```python
from build123d import *

# Parameters (mm, degrees)
SKETCH1_R           = 12.7
SKETCH1_R_2         = 2.4892
BOSS_EXTRUDE1_DEPTH = 0.79375


with BuildPart() as part:
    # Sketch1 → Boss-Extrude1 (new, symmetric)
    with BuildSketch(Plane(origin=(0, 0, 0), x_dir=(0, 0, -1), z_dir=(1, 0, 0))):
        with BuildLine():
            Line((-36.765056818, -4.392675398), (-7.053551136, -16.838589027))
            ThreePointArc((-7.053551136, -16.838589027), (0, -18.25625), (7.053551136, -16.838589027))
            Line((7.053551136, -16.838589027), (36.765056818, -4.392675398))
            ThreePointArc((36.765056818, -4.392675398), (39.6875, 0), (36.765056818, 4.392675398))
            Line((36.765056818, 4.392675398), (7.053551136, 16.838589027))
            ThreePointArc((7.053551136, 16.838589027), (0, 18.25625), (-7.053551136, 16.838589027))
            Line((-7.053551136, 16.838589027), (-36.765056818, 4.392675398))
            ThreePointArc((-36.765056818, 4.392675398), (-39.6875, 0), (-36.765056818, -4.392675398))
        make_face()
        Circle(SKETCH1_R, mode=Mode.SUBTRACT)
        with Locations((34.925, 0)):
            Circle(SKETCH1_R_2, mode=Mode.SUBTRACT)
        with Locations((-34.925, 0)):
            Circle(SKETCH1_R_2, mode=Mode.SUBTRACT)
    extrude(amount=BOSS_EXTRUDE1_DEPTH, both=True)


solid = part.part
```
Input: part model. Units: mm. Frame: model coordinates. Round coordinates to 2 decimals unless told otherwise and drop trailing zeros. Loops run counter-clockwise (first coordinate to the right, second up) from the corner with the lowest first, then second, coordinate; pieces in that order, holes last.
1) Section query C-C on x = -0.3. Return the cut outline in (y, z) (1 decimal), plus the area to 3 significant figures.
Ans:
outline: (-16.8, -7.1) - (-4.4, -36.8) arc R4.8 ccw to (4.4, -36.8) - (16.8, -7.1) arc R18.3 ccw to (16.8, 7.1) - (4.4, 36.8) arc R4.8 ccw to (-4.4, 36.8) - (-16.8, 7.1) arc R18.3 ccw to start; hole circle Ø25.4 at (0, 0); hole circle Ø5 at (0, -34.9); hole circle Ø5 at (0, 34.9)
area: 1,260 mm2
2) Material intervals for line 1 (Z direction, x = -0.2, y = -2); line 2 (Y direction, x = -0.4, z = 0); line 3 (Z direction, x = -0.5, y = -1), sorted ascending.
Ans:
line 1: z = -39.25 to -36.41, -33.44 to -12.54, 12.54 to 33.44, 36.41 to 39.25
line 2: y = -18.26 to -12.7, 12.7 to 18.26
line 3: z = -39.58 to -37.2, -32.65 to -12.66, 12.66 to 32.65, 37.2 to 39.58
3) Pull-direction query (Y, two-part tool) for faces 1 (the cylindrical face through (-0.01, -12.4, 2.75)), 2 (the flat face through (0.011, 10.703, 21.701)), 3 (the cylindrical face through (0.011, -0.078, -39.687)); classes: released by +Y, released by -Y, zero draft, split by the parting line, or undercut.
Ans:
face 1: undercut
face 2: released by +Y
face 3: split by the parting line
4) Pin query (flat end, axial travel): pin 1 (8 mm diameter, centred on y = 2, z = 5, fed in from +X). Return the tip coordinate at first contact, or that it passes through.
Ans:
pin 1: passes through
5) Section query D-D on z = -10. Return the cut outline in (x, y).
Ans:
outline: (-0.79, -15.6) - (0.79, -15.6) - (0.79, -7.83) - (-0.79, -7.83) - close; (-0.79, 7.83) - (0.79, 7.83) - (0.79, 15.6) - (-0.79, 15.6) - close
6) Section query B-B on z = 0. Return the cut outline in (x, y), plus the area to 3 significant figures.
Ans:
outline: (-0.79, -18.26) - (0.79, -18.26) - (0.79, -12.7) - (-0.79, -12.7) - close; (-0.79, 12.7) - (0.79, 12.7) - (0.79, 18.26) - (-0.79, 18.26) - close
area: 17.6 mm2
7) Section query A-A on y = 0. Return the cut outline in (x, z).
Ans:
outline: (-0.79, -39.69) - (0.79, -39.69) - (0.79, -37.41) - (-0.79, -37.41) - close; (-0.79, -32.44) - (0.79, -32.44) - (0.79, -12.7) - (-0.79, -12.7) - close; (-0.79, 12.7) - (0.79, 12.7) - (0.79, 32.44) - (-0.79, 32.44) - close; (-0.79, 37.41) - (0.79, 37.41) - (0.79, 39.69) - (-0.79, 39.69) - close
